from build123d import *

# Parameters (mm, degrees)
F0_R     = 2.25
F0_R_2   = 4.5
F1_DEPTH = 1
F2_R     = 0.5
F0_W     = 12
F0_H     = 2
F3_DEPTH = 0.5
F4_R     = 0.49999
F5_R     = 0.49999


# Not quite as in the source:
# - a fillet or chamfer is up to 0.001 mm smaller than in the source, because OpenCascade refuses the exact size


with BuildPart() as f1:
    # F0 (on Top) → F1 (new body)
    with BuildSketch(Plane.XY):
        with BuildLine():
            ThreePointArc((-2, -1), (-1.7071067812, -1.7071067812), (-1, -2))
            Line((-1, -2), (15, -2))
            ThreePointArc((15, -2), (15.7071067812, -1.7071067812), (16, -1))
            Line((16, -1), (16, 30))
            ThreePointArc((16, 30), (15.7071067812, 30.7071067812), (15, 31))
            Line((15, 31), (13, 31))
            Line((13, 31), (1, 31))
            Line((1, 31), (-1, 31))
            ThreePointArc((-1, 31), (-1.7071067812, 30.7071067812), (-2, 30))
            Line((-2, 30), (-2, -1))
        make_face()
        with Locations((7, 2.95)):
            Circle(F0_R, mode=Mode.SUBTRACT)
        with Locations((7, 16.8)):
            Circle(F0_R_2, mode=Mode.SUBTRACT)
    extrude(amount=F1_DEPTH)

    # F2
    f2_edges = [f1.edges().sort_by_distance(p)[0] for p in [
        (2.5, 16.8, 0),
        (4.75, 2.95, 0),
    ]]
    fillet(f2_edges, radius=F2_R)

    # F0 (on Top) → F3 (join)
    with BuildSketch(Plane.XY):
        with Locations((7, 32)):
            Rectangle(F0_W, F0_H)
    extrude(amount=F3_DEPTH)

    # F4 (radius 0.5 in the source; OpenCascade refuses exactly that, so slightly less here)
    f4_edges = [f1.edges().sort_by_distance(p)[0] for p in [
        (-2, 14.5, 1),
        (-1.707107, -1.707107, 1),
        (7, -2, 1),
        (15.707107, -1.707107, 1),
        (16, 14.5, 1),
        (15.707107, 30.707107, 1),
        (7, 31, 1),
        (-1.707107, 30.707107, 1),
        (4.75, 2.95, 1),
        (2.5, 16.8, 1),
    ]]
    fillet(f4_edges, radius=F4_R)

    # F5 (radius 0.5 in the source; OpenCascade refuses exactly that, so slightly less here)
    f5_edges = [f1.edges().sort_by_distance(p)[0] for p in [
        (1, 32, 0.5),
        (13, 32, 0.5),
    ]]
    fillet(f5_edges, radius=F5_R)


solid = f1.part
Geometry check sheet. Reference: the model listing, model coordinates, mm. A direction names the side the tool comes from. Round coordinates to 2 decimals unless told otherwise and drop trailing zeros. Write each loop counter-clockwise with the first axis right and the second up, starting at its lowest first coordinate (ties: lowest second). Pieces come first, ordered by that corner, then holes.
Item 1: Section check A-A (x = 7). Give the number of separate pieces and of enclosed holes in the cut face, plus the area to 3 significant figures.
Determined:
separate pieces: 3
enclosed holes: 0
area: 20.0 mm2
Item 2: Access from +Z, -Z, +X, -X, +Y, -Y to the whole of each face (thin tool, end or side, straight path). Record for faces 1 (the face through (-1.715, -1.699, 0.247)), 2 (the face through (7, 32, 0.5)).
Determined:
face 1: +Z, -Z, -X, -Y
face 2: +Z, +X, -X, +Y
Item 3: Section check C-C (z = 0.3). Record the boundary of the cut face in (x, y), plus the area to 3 significant figures.
Determined:
outline: (-2, -1) arc R1 ccw to (-1, -2) - (15, -2) arc R1 ccw to (16, -1) - (16, 30) arc R1 ccw to (15, 31) - (12.9, 31) - (12.9, 33) - (1.1, 33) - (1.1, 31) - (-1, 31) arc R1 ccw to (-2, 30) - close; hole circle Ø9.08 at (7, 16.8); hole circle Ø4.58 at (7, 2.95)
area: 535 mm2
Item 4: Material ranges on line 1 along Y through (x, z) = (7, 0.55); line 2 along Y through (x, z) = (5.5, 0.7); line 3 along Y through (x, z) = (3, 0.85), recorded low to high.
Determined:
line 1: y = -2 to 0.7, 5.2 to 12.3, 21.3 to 31
line 2: y = -1.96 to 1.22, 4.68 to 12.51, 21.09 to 30.96
line 3: y = -1.86 to 14.44, 19.16 to 30.86
Item 5: Go/stop test with a flat-tipped pin: pin 1 Ø6 at (x, y) = (2.5, 3) entering from -Z. Record where the tip stops, or that it passes through.
Determined:
pin 1: stops at z = 0
